Model file for the job. Use its own axes, mm. A direction names the side the tool comes from. Round coordinates to 2 decimals unless told otherwise and drop trailing zeros. Order: outer loops, then holes, each group sorted by start corner. A loop starts at its lowest first (then second) coordinate and runs counter-clockwise, first axis right, second up. Notation, with made-up numbers: (-29, -32.5) - (-8, -32.5) arc R9 cw to (-8, -16.5) - close; hole circle Ø8 at (-10, 13). An arc over 180 degrees is marked (long way). Write item = value, one per line.
```python
from build123d import *

# Parameters (mm, degrees)
SKETCH1_R               = 2.1828125
BOSS_EXTRUDE1_DEPTH     = 9.525
CUT_EXTRUDE1_DEPTH      = 25.490757185
CUT_EXTRUDE1_DEPTH_BACK = 25.490757185
SKETCH2_R               = 2.1828125
FILLET1_R               = 4.7625
FILLET2_R               = 3.175
CHAMFER1_SIZE           = 0.396875


with BuildPart() as part:
    # Sketch1 → Boss-Extrude1 (new body)
    with BuildSketch(Plane(origin=(0, 0, 0), x_dir=(1, 0, 0), z_dir=(0, 1, 0))):
        with BuildLine():
            Line((-4.7625, 0), (-4.7625, -9.525))
            Line((-4.7625, -9.525), (-17.4625, -9.525))
            Line((-17.4625, -9.525), (-17.4625, -12.7))
            Line((-17.4625, -12.7), (17.4625, -12.7))
            Line((17.4625, -12.7), (17.4625, -9.525))
            Line((17.4625, -9.525), (4.7625, -9.525))
            Line((4.7625, -9.525), (4.7625, 0))
            ThreePointArc((4.7625, 0), (0, 4.7625), (-4.7625, 0))
        make_face()
        with Locations(Location((0, 0, 0), (0, 0, 90))):
            Circle(SKETCH1_R, mode=Mode.SUBTRACT)
    extrude(amount=BOSS_EXTRUDE1_DEPTH)

    # Sketch2 → Cut-Extrude1 (cut, two sides: drawn at the far end of the back side and taken through both)
    with BuildSketch(Plane(origin=(0, 0, 9.525), x_dir=(-1, 0, 0), z_dir=(0, 0, -1)).offset(-CUT_EXTRUDE1_DEPTH_BACK)):
        with Locations((-12.7, 4.7625)):
            Circle(SKETCH2_R)
        with Locations((12.7, 4.7625)):
            Circle(SKETCH2_R)
    extrude(amount=CUT_EXTRUDE1_DEPTH + CUT_EXTRUDE1_DEPTH_BACK, mode=Mode.SUBTRACT)

    # Fillet1
    fillet1_edges = [part.edges().sort_by_distance(p)[0] for p in [
        (17.4625, 9.525, 11.1125),
        (17.4625, 0, 11.1125),
        (-17.4625, 9.525, 11.1125),
        (-17.4625, 0, 11.1125),
    ]]
    fillet(fillet1_edges, radius=FILLET1_R - 0.0001)  # a hair under: the kernel refuses the full size

    # Fillet2
    fillet2_edges = [part.edges().sort_by_distance(p)[0] for p in [
        (4.7625, 4.7625, 9.525),
        (-4.7625, 4.7625, 9.525),
    ]]
    fillet(fillet2_edges, radius=FILLET2_R)

    # Chamfer1
    chamfer1_edges = [part.edges().sort_by_distance(p)[0] for p in [
        (-4.7625, 0, 3.175),
        (0, 0, -4.7625),
        (0, 0, 2.1828125),
        (14.8828125, 4.7625, 12.7),
        (14.8828125, 4.7625, 9.525),
        (-10.5171875, 4.7625, 12.7),
        (-10.5171875, 4.7625, 9.525),
        (0, 9.525, 12.7),
        (10.3188, 9.525, 9.525),
        (10.3188, 0, 9.525),
        (16.067625335, 1.394874665, 9.525),
        (16.067625335, 8.130125335, 9.525),
        (0, 0, 12.7),
        (-16.067625335, 1.394874665, 12.7),
        (-16.067625335, 8.130125335, 12.7),
        (16.067625335, 1.394874665, 12.7),
        (16.067625335, 8.130125335, 12.7),
        (-16.067625335, 1.394874665, 9.525),
        (-16.067625335, 8.130125335, 9.525),
        (0, 9.525, -4.7625),
        (4.7625, 0, 3.175),
        (4.7625, 9.525, 3.175),
        (-10.3188, 9.525, 9.525),
        (-10.3188, 0, 9.525),
        (5.69243597, 0, 8.59506403),
        (5.69243597, 9.525, 8.59506403),
        (-5.69243597, 0, 8.59506403),
        (-5.69243597, 9.525, 8.59506403),
        (-4.7625, 9.525, 3.175),
    ]]
    chamfer(chamfer1_edges, length=CHAMFER1_SIZE)


solid = part.part
```
1) Wall check: line 1 along X through (y, z) = (7.25, 0); line 2 along Y through (x, z) = (12.7, 10.5) (3 decimals); line 3 along X through (y, z) = (4.25, 11.75). Give the ranges that are in metal, low to high.
Conclusion:
line_1 = -4.76 to -2.18, 2.18 to 4.76
line_2 = 0 to 2.58, 6.945 to 9.525
line_3 = -17.43 to -14.82, -10.58 to 10.58, 14.82 to 17.43
2) Cut at C-C (y = 3.75). Give the number of separate pieces and of enclosed holes in the cut face, and give its area (3 significant figures).
Conclusion:
separate_pieces = 3
enclosed_holes = 1
area = 200 mm^2
3) Cut at A-A (x = 0). Write the cut outline in (y, z) (1 decimal), and give its area (3 significant figures).
Conclusion:
outline = (0, -4.4) - (0.4, -4.8) - (9.1, -4.8) - (9.5, -4.4) - (9.5, -2.2) - (0.4, -2.2) - (0, -2.6) - close; (0, 2.6) - (0.4, 2.2) - (9.5, 2.2) - (9.5, 12.3) - (9.1, 12.7) - (0.4, 12.7) - (0, 12.3) - close
area = 124 mm^2
4) Mould opens along Y. For faces 4 (the face through (5.59, 9.24, 8.65)), 5 (the face through (5.642, 0.289, 8.696)), 6 (the face through (-10.97, 3.43, 11.13)) say: +Y half, -Y half, draft (parallel to the pull), parting line (faces both ways), or undercut.
Conclusion:
face_4 = +Y half
face_5 = -Y half
face_6 = undercut
5) Flat gauge pins, fed straight in: pin 1 Ø2.5 at (x, z) = (0, 0) entering from -Y; pin 2 Ø2.5 at (x, y) = (-14, 4) entering from -Z (3 decimals); pin 3 Ø4 at (y, z) = (3, -2) entering from -X; pin 4 Ø3 at (y, z) = (6, 4.5) entering from +X. Where does each tip first touch, or does it go through?
Conclusion:
pin_1 = through
pin_2 = 9.525
pin_3 = -4.76
pin_4 = 4.76
6) 3-axis set-ups, long thin cutter, end or side, ignore diameter. For faces 1 (the face through (15.898, 1.634, 9.632)), 2 (the face through (-4.762, 5, 3)), 3 (the face through (11, 7, 9.525)): which of +Z, -Z, +X, -X, +Y, -Y reach the whole face in a straight line?
Conclusion:
face_1 = -Z, +X, -Y
face_2 = -Z, -X, +Y, -Y
face_3 = -Z, +X, +Y, -Y
7) Cut at B-B (z = 5.5). Write the cut outline in (x, y) (1 decimal), and give its area (3 significant figures).
Conclusion:
outline = (-4.8, 0.4) - (-4.4, 0) - (4.4, 0) - (4.8, 0.4) - (4.8, 9.1) - (4.4, 9.5) - (-4.4, 9.5) - (-4.8, 9.1) - close
area = 90.4 mm^2
